Can you work these out from the model? Positions are in its coordinate system, mm. A direction names the side the tool comes from. Round coordinates to 2 decimals unless told otherwise and drop trailing zeros. Loops run counter-clockwise (first coordinate to the right, second up) from the corner with the lowest first, then second, coordinate; pieces in that order, holes last.
(1) I want a section at A-A on x = -25. Write out the boundary of the cut face in (y, z), plus the area to 3 significant figures.
(2) Will these pins go through, and if not, where does the flat tip stop? pin 1 Ø2.5 at (x, z) = (-13.42, -7.75) entering from +Y; pin 2 Ø1 at (x, y) = (4.5, 18.5) entering from +Z; pin 3 Ø2 at (y, z) = (23, -3.5) entering from -X; pin 4 Ø12 at (x, y) = (-16, 11) entering from -Z.
(3) Thinking about a two-plate mould opening in Z: for faces 1 (the face through (27.003, 28.028, -0.631)), 2 (the face through (19.94, 12.82, -0.65)), 3 (the face through (29.9, 28, 0)), which applies, released by +Z, released by -Z, zero draft, split by the parting line, or undercut?
(4) If I drill on line 1 along X through (y, z) = (27.1, 0); line 2 along Z through (x, y) = (-25, 28.3); line 3 along Z through (x, y) = (0, 25), over which ranges is the centre line in solid material (lowest first)?
(5) I want a section at C-C on y = 16.75. Write out the boundary of the cut face in (x, z).
(6) I want a section at B-B on x = -7. Write out the boundary of the cut face in (y, z).
(7) Which directions (+Z, -Z, +X, -X, +Y, -Y) give clear straight access to the entire face, cutting with the end or side of a thin tool? Please do faces 4 (the face through (-19.575, 13.182, -13.797)), 5 (the face through (-11.96, 2.96, -3.8)).
(8) I want a section at D-D on x = 6.5. Write out the boundary of the cut face in (y, z).
Autodesk Inventor part; units mm, degrees
ref_plane "YZ Plane" through (0, 0, 0) normal (1, 0, 0) x (0, 1, 0)
ref_plane "XZ Plane" through (0, 0, 0) normal (0, 1, 0) x (-1, 0, 0)
ref_plane "XY Plane" through (0, 0, 0) normal (0, 0, 1) x (1, 0, 0)
sketch "Sketch1" plane through (0, 0, 0) normal (0, 1, 0) x (-1, 0, 0)
  circle A0 centre (0, 0) radius 19.95
  dimension "d0" = 39.9
extrude "Extrusion1" add sketch "Sketch1" along normal blind 6
sketch "Sketch2" plane through (0, 6, 0) normal (0, 1, 0) x (1, 0, 0)
  circle A0 centre (0, 0) radius 19.95
  circle A1 centre (0, 0) radius 18.75
  dimension "d3" = 37.5
  dimension "d4" = 39.9
extrude "Extrusion2" add sketch "Sketch2" along normal blind 20
sketch "Sketch3" plane through (0, 0, 0) normal (0, -1, 0) x (1, 0, 0)
  circle A0 centre (-7, 0) radius 6.25
  circle A1 centre (0, -15.5) radius 1.6
  circle A2 centre (13.4234, -7.75) radius 1.6
  circle A3 centre (13.4234, 7.75) radius 1.6
  circle A4 centre (0, 15.5) radius 1.6
  circle A5 centre (-13.4234, 7.75) radius 1.6
  circle A6 centre (-13.4234, -7.75) radius 1.6
  point P0 (0, 0)
  dimension "d7" = 0
  dimension "d8" = 7
  dimension "d9" = 12.5
  dimension "d10" = 3.2
  dimension "d11" = 0
  dimension "d12" = 15.5
  dimension "d15" = 360
extrude "Extrusion3" cut sketch "Sketch3" against normal up to next
sketch "Sketch4" plane through (0, 26, 0) normal (0, 1, 0) x (1, 0, 0)
  circle A0 centre (0, 0) radius 18.75
  line L0 (-29.9, -20.9) -> (29.9, -20.9)
  line L1 (29.9, -20.9) -> (29.9, 20.9)
  line L2 (29.9, 20.9) -> (-29.9, 20.9)
  line L3 (-29.9, 20.9) -> (-29.9, -20.9)
  line L4 (-29.9, -20.9) -> (29.9, 20.9) construction
  line L5 (29.9, -20.9) -> (-29.9, 20.9) construction
  dimension "d19" = 59.8
  dimension "d20" = 41.8
extrude "Extrusion4" add sketch "Sketch4" along normal blind 4
sketch "Sketch5" plane through (0, 30, 0) normal (0, 1, 0) x (1, 0, 0)
  line L0 (29.9, -20.9) -> (29.9, 20.9)
  line L1 (-29.9, 20.9) -> (-29.9, -20.9)
  circle A0 centre (25, 15) radius 2.1
  circle A1 centre (25, 0) radius 2.1
  circle A2 centre (25, -15) radius 2.1
  circle A3 centre (-25, 15) radius 2.1
  circle A4 centre (-25, 0) radius 2.1
  circle A5 centre (-25, -15) radius 2.1
  point P0 (0, 0)
  dimension "d23" = 0
  dimension "d24" = 25
  dimension "d25" = 15
  dimension "d26" = 25
  dimension "d27" = 25
  dimension "d28" = 15
  dimension "d29" = 4.2
  dimension "d30" = 4.2
  dimension "d31" = 4.2
  dimension "d33" = 0
  dimension "d34" = 15
  dimension "d35" = 15
  dimension "d36" = 25
  dimension "d37" = 25
  dimension "d38" = 25
  dimension "d39" = 4.2
  dimension "d40" = 4.2
  dimension "d41" = 4.2
extrude "Extrusion5" cut sketch "Sketch5" against normal up to next
sketch "Sketch7" plane through (0, 26, 0) normal (0, -1, 0) x (1, 0, 0)
  line L0 (29.9, -20.9) -> (-29.9, -20.9)
  line L1 (14.3023, -9.9973) -> (16.3514, -11.4296)
  line L2 (-29.9, 20.9) -> (29.9, 20.9)
  line L3 (14.3023, 9.9973) -> (16.3514, 11.4296)
  circle A0 centre (0, 0) radius 19.95
  arc A1 (18.3028, 7.9379) -> (13.7426, 14.4618) centre (16.3514, 11.4296) ccw
  arc A2 (13.7426, -14.4618) -> (18.3028, -7.9379) centre (16.3514, -11.4296) ccw
  arc A3 (-13.7426, 14.4618) -> (-18.3028, 7.9379) centre (-16.3514, 11.4296) ccw
  arc A4 (-18.3028, -7.9379) -> (-13.7426, -14.4618) centre (-16.3514, -11.4296) ccw
  line L4 (-16.3514, 11.4296) -> (-14.3023, 9.9973)
  line L5 (-14.3023, -9.9973) -> (-16.3514, -11.4296)
  dimension "d48" = 8
  dimension "d49" = 8
  dimension "d50" = 8
  dimension "d51" = 8
  dimension "d52" = 32.7028
  dimension "d53" = 32.7028
  dimension "d54" = 22.8591
extrude "Extrusion8" add sketch "Sketch7" along normal blind 26 contours A0 A3 | A4 A0
properties part number "motorHolder57mmVer2" material "ABS Plastic"
Filled sheet:
1. outline: (26, -20.9) - (30, -20.9) - (30, -17.1) - (26, -17.1) - close; (26, -12.9) - (30, -12.9) - (30, -2.1) - (26, -2.1) - close; (26, 2.1) - (30, 2.1) - (30, 12.9) - (26, 12.9) - close; (26, 17.1) - (30, 17.1) - (30, 20.9) - (26, 20.9) - close
1. area: 117 mm2
2. pin 1: passes through
2. pin 2: stops at z = 19.54
2. pin 3: stops at x = -19.79
2. pin 4: stops at z = -17.26
3. face 1: undercut
3. face 2: split by the parting line
3. face 3: zero draft
4. line 1: x = -29.9 to -27.1, -22.9 to -18.75, 18.75 to 22.9, 27.1 to 29.9
4. line 2: z = -20.9 to -17.1, -12.9 to -2.1, 2.1 to 12.9, 17.1 to 20.9
4. line 3: z = -19.95 to -18.75, 18.75 to 19.95
5. outline: (-18.3, -7.94) arc R4 ccw (long way) to (-13.74, -14.46) arc R19.95 ccw (long way) to (-13.74, 14.46) arc R4 ccw (long way) to (-18.3, 7.94) arc R19.95 ccw to start; hole circle Ø37.5 at (0, 0)
6. outline: (0, -18.68) - (26, -18.68) - (26, -20.9) - (30, -20.9) - (30, -17.39) - (6, -17.39) - (6, -6.25) - (0, -6.25) - close; (0, 6.25) - (6, 6.25) - (6, 17.39) - (30, 17.39) - (30, 20.9) - (26, 20.9) - (26, 18.68) - (0, 18.68) - close
7. face 4: -Y
7. face 5: +Y, -Y
8. outline: (0, -18.86) - (26, -18.86) - (26, -20.9) - (30, -20.9) - (30, -17.59) - (6, -17.59) - (6, 17.59) - (30, 17.59) - (30, 20.9) - (26, 20.9) - (26, 18.86) - (0, 18.86) - close
